```python
from build123d import *

# Parameters (mm, degrees)
SKETCH1_W           = 54.864
SKETCH1_H           = 35.56
BOSS_EXTRUDE1_DEPTH = 3.81
SKETCH2_R           = 2.1717
SKETCH2_W           = 39.624
SKETCH2_H           = 20.32
CUT_EXTRUDE2_DEPTH  = 3.81
SKETCH3_W           = 6.35
SKETCH3_H           = 6.352840925
SKETCH3_H_2         = 6.35
BOSS_EXTRUDE2_DEPTH = 30.48
SKETCH4_R           = 2.1717
CUT_EXTRUDE3_DEPTH  = 6.35


with BuildPart() as part:
    # Sketch1 → Boss-Extrude1 (new body)
    with BuildSketch(Plane(origin=(0, 0, 0), x_dir=(1, 0, 0), z_dir=(0, 1, 0))):
        with Locations((2.806390244, -14.88997561)):
            Rectangle(SKETCH1_W, SKETCH1_H)
    extrude(amount=BOSS_EXTRUDE1_DEPTH)

    # Sketch2 → Cut-Extrude2 (cut)
    with BuildSketch(Plane(origin=(0, 3.81, 0), x_dir=(1, 0, 0), z_dir=(0, 1, 0))):
        with Locations(Location((-20.815609756, -0.91997561, 0), (0, 0, 270))):
            Circle(SKETCH2_R)
        with Locations(Location((-20.815609756, -19.96997561, 0), (0, 0, 270))):
            Circle(SKETCH2_R)
        with Locations(Location((26.428390244, -19.96997561, 0), (0, 0, 270))):
            Circle(SKETCH2_R)
        with Locations(Location((26.428390244, -0.91997561, 0), (0, 0, 270))):
            Circle(SKETCH2_R)
        with Locations((2.806390244, -14.88997561)):
            Rectangle(SKETCH2_W, SKETCH2_H)
    extrude(amount=-CUT_EXTRUDE2_DEPTH, mode=Mode.SUBTRACT)

    # Sketch3 → Boss-Extrude2 (add)
    with BuildSketch(Plane(origin=(0, 3.81, 0), x_dir=(1, 0, 0), z_dir=(0, 1, 0))):
        with Locations((-21.450609756, -29.493555148)):
            Rectangle(SKETCH3_W, SKETCH3_H)
        with Locations((27.063390244, -29.49497561)):
            Rectangle(SKETCH3_W, SKETCH3_H_2)
    extrude(amount=BOSS_EXTRUDE2_DEPTH)

    # Sketch4 → Cut-Extrude3 (cut)
    with BuildSketch(Plane.XY.offset(32.66997561)):
        with Locations((-21.831609756, 30.988)):
            Circle(SKETCH4_R)
        with Locations((-21.831609756, 20.955)):
            Circle(SKETCH4_R)
        with Locations((27.444390244, 30.988)):
            Circle(SKETCH4_R)
        with Locations((27.444390244, 20.955)):
            Circle(SKETCH4_R)
    extrude(amount=-CUT_EXTRUDE3_DEPTH, mode=Mode.SUBTRACT)


solid = part.part
```
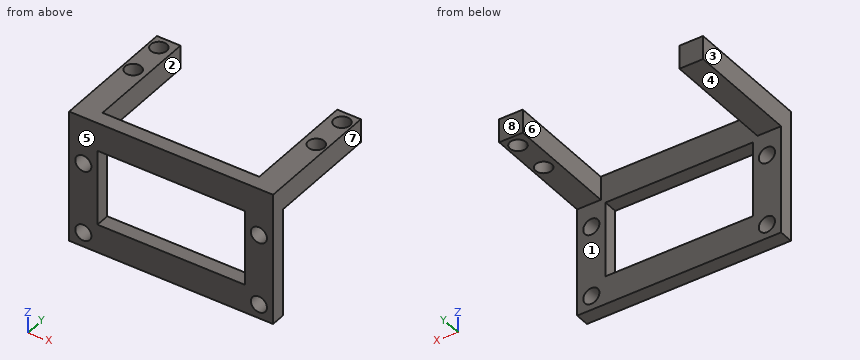
Can you work these out from the model? Positions are in its coordinate system, mm. Face numbers are marked on the shaded views. A direction names the side the tool comes from. Give positions to 0.01 mm unless a question says otherwise; leave off trailing zeros. Loops run counter-clockwise (first coordinate to the right, second up) from the corner with the lowest first, then second, coordinate; pieces in that order, holes last. Notation, with made-up numbers: M 42.5,62.25 L 61.5,62.25 A7 ccw 61.5,67.25 Z; hole C 3,-34 d1. An arc over 180 degrees is marked long. One line per question, with ' | ' between items. Start each with the question number.
Q1. For the marked faces 1, 2, 3, 4 and 5, which set-ups out of +Z, -Z, +X, -X, +Y, -Y let a thin tool reach every point of the face, with its end or its side?
Q2. If we mould it in two halves opening along X, with no side actions, what happens to the marked faces 6, 7 and 8? For each: +X half, -X half, draft (parallel to the pull), parting line (faces both ways), or undercut.
Q3. If we section it at A-A (x = 15): Please give me the cut outline in (y, z).
Q4. If I drill on line 1 (X direction, y = 8, z = 27.5); line 2 (X direction, y = 2, z = 9); line 3 (Y direction, x = 17, z = 31.5), over which ranges is the centre line in solid material (lowest first)? Write a range as from..to.
Q5. If we section it at B-B (z = 14.5): Please give me the cut outline in (x, y), plus the area to 3 significant figures.
Q6. If we section it at C-C (y = 32.5): Please give me the cut outline in (x, z), plus the area to 3 significant figures.
Q7. If we section it at D-D (z = 21): Please give me the cut outline in (x, y), plus the area to 3 significant figures.
Q8. For pin 1 Ø10 at (x, z) = (20.5, 21.5) entering from -Y; pin 2 Ø5 at (x, y) = (28.5, 17.5) entering from -Z; pin 3 Ø5 at (x, z) = (-20.82, 19.97) entering from +Y; pin 4 Ø1.3 at (x, y) = (-21.5, 31) entering from +Z, each with a flat end and sliding along its axis, tell me the tip position at first contact or that it passes through.
Computed:
1) face 1: -Z, +Y | face 2: +Z, -Z, +Y | face 3: +Z, -Z, -X, +Y, -Y | face 4: -Z, +X, -X, +Y | face 5: +Z, -Z, +X, -X, -Y
2) face 6: undercut | face 7: +X half | face 8: draft
3) outline: M 0,-2.89 L 3.81,-2.89 L 3.81,4.73 L 0,4.73 Z; M 0,25.05 L 3.81,25.05 L 3.81,32.67 L 0,32.67 Z
4) line 1: x = -24.63..-18.28, 23.89..30.24 | line 2: x = -24.63..-17.01, 22.62..30.24 | line 3: y = 0..3.81
5) outline: M -24.63,0 L -17.01,0 L -17.01,3.81 L -24.63,3.81 Z; M 22.62,0 L 30.24,0 L 30.24,3.81 L 22.62,3.81 Z | area: 58.1 mm²
6) outline: M -24.63,26.32 L -18.28,26.32 L -18.28,32.67 L -20.27,32.67 L -20.27,26.32 L -23.39,26.32 L -23.39,32.67 L -24.63,32.67 Z; M 23.89,26.32 L 25.89,26.32 L 25.89,32.67 L 23.89,32.67 Z; M 29,26.32 L 30.24,26.32 L 30.24,32.67 L 29,32.67 Z | area: 41.1 mm²
7) outline: M -24.63,0 L -22.73,0 L -22.73,3.81 L -24.63,3.81 Z; M -18.9,0 L -17.01,0 L -17.01,3.81 L -18.9,3.81 Z; M 22.62,0 L 24.52,0 L 24.52,3.81 L 22.62,3.81 Z; M 28.34,0 L 30.24,0 L 30.24,3.81 L 28.34,3.81 Z | area: 28.9 mm²
8) pin 1: stops at y = 0 | pin 2: stops at z = 26.32 | pin 3: stops at y = 3.81 | pin 4: stops at z = 26.32
